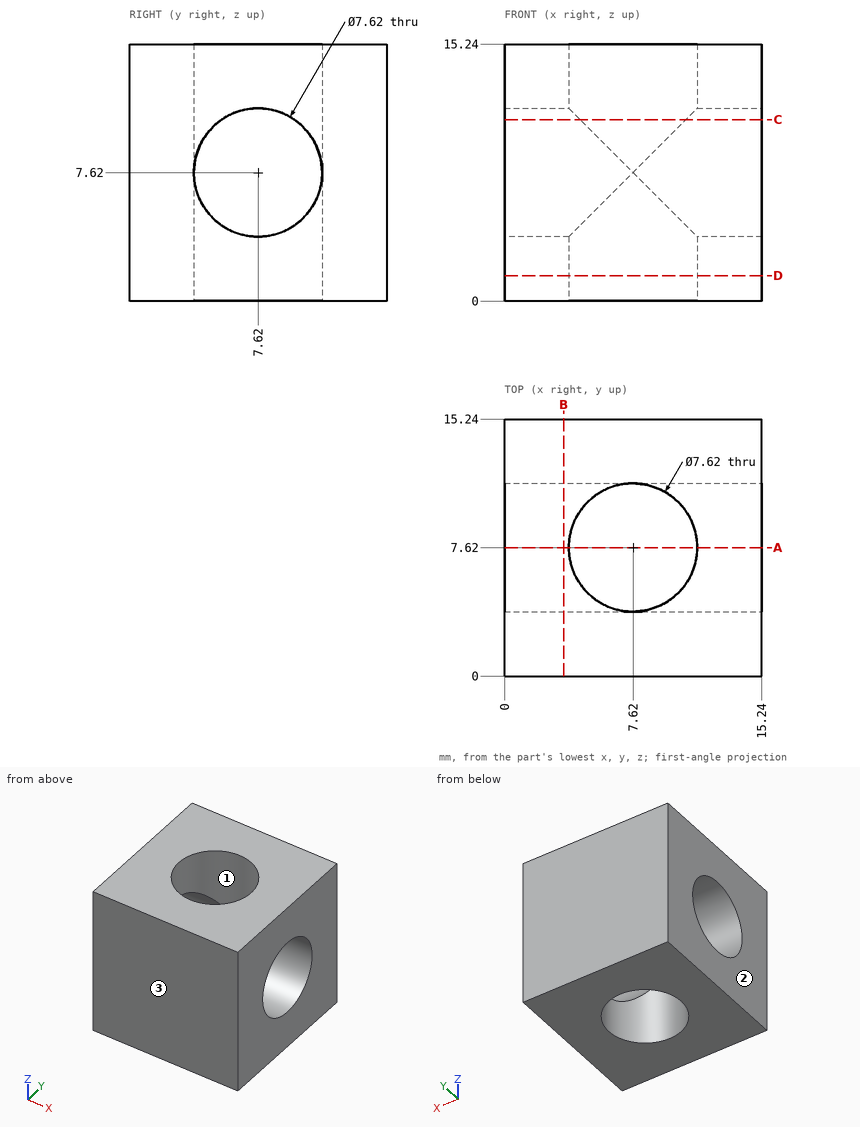
Job drawing, mm, ordinate dimensions from the low corner. One solid piece. Round coordinates to 2 decimals unless told otherwise and drop trailing zeros. Loops run counter-clockwise (first coordinate to the right, second up) from the corner with the lowest first, then second, coordinate; pieces in that order, holes last. Notation, with made-up numbers: (-11.5, 77.25) -> (-4.5, 77.25) arc R12 cw to (-4.5, 94.25) -> close; hole circle Ø5 at (65.25, 4). An arc over 180 degrees is marked (long way). One line per item, written item: value. Start each with the question number.
Q1. Cut at B-B on x = 3.5. List the corners of the cut face in (y, z).
Q2. Probe line 1 along Y through (x, z) = (7.62, 6); line 2 along X through (y, z) = (10.75, 1.25); line 3 along Y through (x, z) = (1.25, 9). List the from-to ranges inside material, lowest first.
Q3. Two-plate mould, pull along Y, no slides. Class the marked faces 1, 2 and 3: released by +Y, released by -Y, zero draft, split by the parting line, or undercut.
Q4. Cut at A-A on y = 7.62. List the corners of the cut face in (x, z), plus the area to 3 significant figures.
Q5. Cut at C-C on z = 10.75. List the corners of the cut face in (x, y).
Computed:
1. outline: (0, 0) -> (15.24, 0) -> (15.24, 15.24) -> (0, 15.24) -> close; hole circle Ø7.62 at (7.62, 7.62)
2. line 1: 0 to 3.81, 11.43 to 15.24
2. line 2: 0 to 5.45, 9.79 to 15.24
2. line 3: 0 to 4.07, 11.17 to 15.24
3. face 1: undercut
3. face 2: zero draft
3. face 3: released by -Y
4. outline: (0, 0) -> (3.81, 0) -> (3.81, 3.81) -> (0, 3.81) -> close; (0, 11.43) -> (3.81, 11.43) -> (3.81, 15.24) -> (0, 15.24) -> close; (11.43, 0) -> (15.24, 0) -> (15.24, 3.81) -> (11.43, 3.81) -> close; (11.43, 11.43) -> (15.24, 11.43) -> (15.24, 15.24) -> (11.43, 15.24) -> close
4. area: 58.1 mm²
5. outline: (0, 0) -> (15.24, 0) -> (15.24, 5.45) -> (10.75, 5.45) arc R3.81 cw to (4.49, 5.45) -> (0, 5.45) -> close; (0, 9.79) -> (4.49, 9.79) arc R3.81 cw to (10.75, 9.79) -> (15.24, 9.79) -> (15.24, 15.24) -> (0, 15.24) -> close
